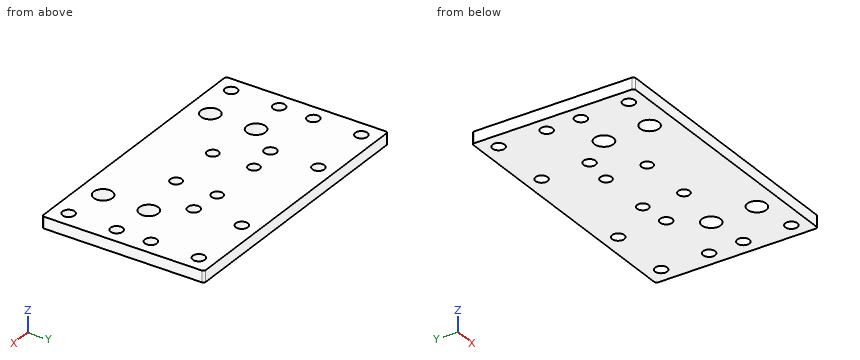
from build123d import *

# Parameters (mm, degrees)
SKETCH1_W               = 120
SKETCH1_H               = 71
SKETCH1_R               = 2.5
BOSS_EXTRUDE1_DEPTH     = 5
FILLET1_R               = 1
SKETCH3_R               = 2.65
SKETCH3_R_2             = 4.1275
CUT_EXTRUDE1_DEPTH      = 39
CUT_EXTRUDE1_DEPTH_BACK = 46


with BuildPart() as part:
    # Sketch1 → Boss-Extrude1 (new body)
    with BuildSketch(Plane.XY):
        with Locations((60, 35.5)):
            Rectangle(SKETCH1_W, SKETCH1_H)
        with Locations((48, 44.5)):
            Circle(SKETCH1_R, mode=Mode.SUBTRACT)
        with Locations((72, 44.5)):
            Circle(SKETCH1_R, mode=Mode.SUBTRACT)
        with Locations((48, 26.5)):
            Circle(SKETCH1_R, mode=Mode.SUBTRACT)
        with Locations((72, 26.5)):
            Circle(SKETCH1_R, mode=Mode.SUBTRACT)
    extrude(amount=BOSS_EXTRUDE1_DEPTH)

    # Fillet1
    fillet1_edges = [part.edges().sort_by_distance(p)[0] for p in [
        (0, 71, 2.5),
        (120, 71, 2.5),
        (120, 0, 2.5),
        (0, 0, 2.5),
    ]]
    fillet(fillet1_edges, radius=FILLET1_R)

    # Sketch3 → Cut-Extrude1 (cut, two sides)
    with BuildSketch(Plane(origin=(0, 0, 0), x_dir=(-1, 0, 0), z_dir=(0, 0, -1))) as cut_extrude1_sk:
        with Locations((-113, 64)):
            Circle(SKETCH3_R)
        with Locations((-113, 43)):
            Circle(SKETCH3_R)
        with Locations((-85, 64)):
            Circle(SKETCH3_R)
        with Locations((-113, 28)):
            Circle(SKETCH3_R)
        with Locations((-113, 7)):
            Circle(SKETCH3_R)
        with Locations((-7, 7)):
            Circle(SKETCH3_R)
        with Locations((-7, 28)):
            Circle(SKETCH3_R)
        with Locations((-7, 64)):
            Circle(SKETCH3_R)
        with Locations((-7, 43)):
            Circle(SKETCH3_R)
        with Locations((-35, 64)):
            Circle(SKETCH3_R)
        with Locations((-35, 43)):
            Circle(SKETCH3_R)
        with Locations((-85, 43)):
            Circle(SKETCH3_R)
        with Locations((-25, 30)):
            Circle(SKETCH3_R_2)
        with Locations((-25, 10)):
            Circle(SKETCH3_R_2)
        with Locations((-95, 10)):
            Circle(SKETCH3_R_2)
        with Locations((-95, 30)):
            Circle(SKETCH3_R_2)
    extrude(amount=CUT_EXTRUDE1_DEPTH, mode=Mode.SUBTRACT)
    extrude(cut_extrude1_sk.sketch, amount=-CUT_EXTRUDE1_DEPTH_BACK, mode=Mode.SUBTRACT)


solid = part.part
The model under review builds one solid part; all positions refer to its coordinate system, in mm. Coordinates: 2 decimals unless noted, no trailing zeros. Write each loop counter-clockwise with the first axis right and the second up, starting at its lowest first coordinate (ties: lowest second). Pieces come first, ordered by that corner, then holes. Notation, with made-up numbers: (13.5, 46.25) - (57.5, 46.25) arc R18 cw to (57.5, 66.25) - close; hole circle Ø2 at (5.25, 50). An arc over 180 degrees is marked (long way). Answer as a JSON object with one key per item and string values. Group by question number.
1. Add section B-B (z = 2.05). Give the number of separate pieces and of enclosed holes in the cut face, plus the area to 3 significant figures.
2. Add section D-D (x = 72). Give the boundary of the cut face in (y, z), plus the area to 3 significant figures.
3. Clearance check with a flat-ended pin moving along its axis: pin 1 Ø6 at (x, y) = (113, 7) entering from -Z. State where the tip first meets the part, or that it passes through.
4. To check wall thickness, follow probe 1 along Y at (x, z) = (48, 2.15); probe 2 along Y at (x, z) = (113, 2.3); probe 3 along X at (y, z) = (31, 1.85). State the ranges of each line that lie inside material, in increasing order.
5. Add section A-A (x = 35). Give the boundary of the cut face in (y, z).
6. Add section C-C (y = 64). Give the boundary of the cut face in (x, z).
Findings:
{
 "1": {"separate pieces": "1", "enclosed holes": "20", "area": "7,960 mm²"},
 "2": {"outline": "(0, 0) - (24, 0) - (24, 5) - (0, 5) - close; (29, 0) - (42, 0) - (42, 5) - (29, 5) - close; (47, 0) - (71, 0) - (71, 5) - (47, 5) - close", "area": "305 mm²"},
 "3": {"pin 1": "z = 0"},
 "4": {"probe 1": "0 to 24, 29 to 42, 47 to 71", "probe 2": "0 to 4.35, 9.65 to 25.35, 30.65 to 40.35, 45.65 to 61.35, 66.65 to 71", "probe 3": "0 to 21, 29 to 91, 99 to 120"},
 "5": {"outline": "(0, 0) - (40.35, 0) - (40.35, 5) - (0, 5) - close; (45.65, 0) - (61.35, 0) - (61.35, 5) - (45.65, 5) - close; (66.65, 0) - (71, 0) - (71, 5) - (66.65, 5) - close"},
 "6": {"outline": "(0, 0) - (4.35, 0) - (4.35, 5) - (0, 5) - close; (9.65, 0) - (32.35, 0) - (32.35, 5) - (9.65, 5) - close; (37.65, 0) - (82.35, 0) - (82.35, 5) - (37.65, 5) - close; (87.65, 0) - (110.35, 0) - (110.35, 5) - (87.65, 5) - close; (115.65, 0) - (120, 0) - (120, 5) - (115.65, 5) - close"}
}
